Answer from the drawing. Dimensions are ordinates in mm from the lowest x, y and z of the part. Round coordinates to 2 decimals unless told otherwise and drop trailing zeros. Order: outer loops, then holes, each group sorted by start corner. A loop starts at its lowest first (then second) coordinate and runs counter-clockwise, first axis right, second up.
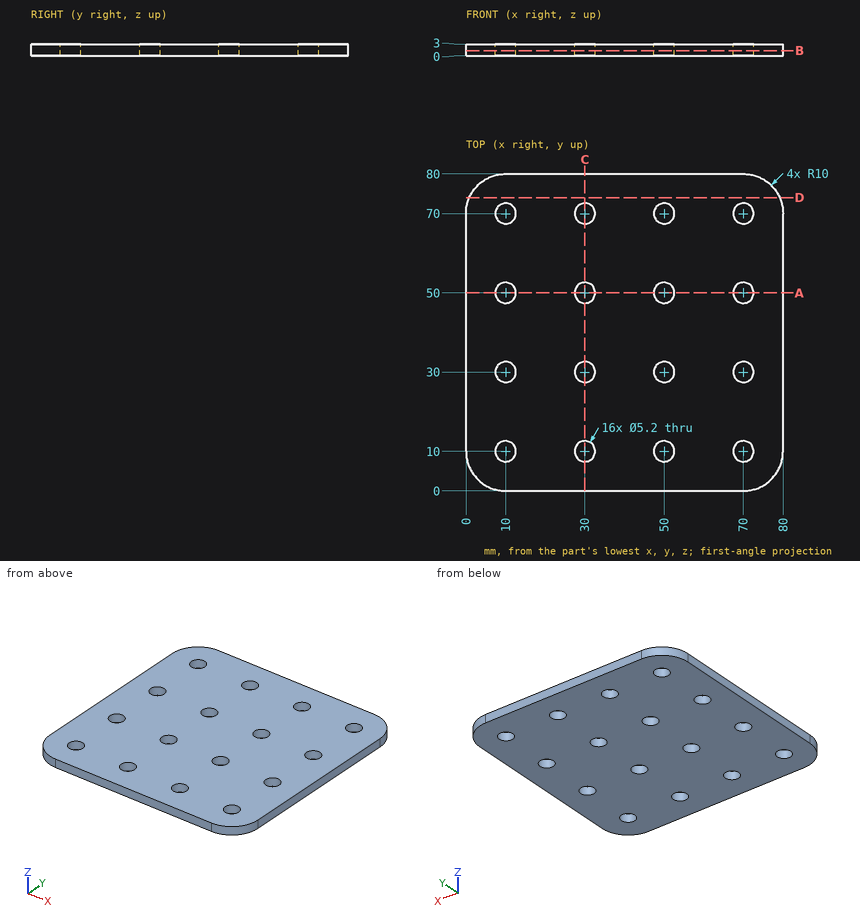
Q1. Straight lines are drawn through the part: probe 1 along Y at (x, z) = (50, 2.35); probe 2 along X at (y, z) = (31, 0.5). For each, find the intervals that lie inside material, in ascending order.
Outcome:
probe 1: y = 0 to 7.4, 12.6 to 27.4, 32.6 to 47.4, 52.6 to 67.4, 72.6 to 80
probe 2: x = 0 to 7.6, 12.4 to 27.6, 32.4 to 47.6, 52.4 to 67.6, 72.4 to 80
Q2. Flat-ended cylindrical pins translate along their axes: pin 1 (7 mm diameter, centred on x = 30, y = 30, fed in from -Z); pin 2 (3 mm diameter, centred on x = 10, y = 70, fed in from +Z) (3 decimals). Find the tip coordinate at first contact, or state that the pin passes through.
Outcome:
pin 1: stops at z = 0
pin 2: passes through
Q3. A cutting plane is placed at A-A, the plane y = 50. Give the vertices of the cut face in (x, z), plus the area to 3 significant figures.
Outcome:
outline: (0, 0) - (7.4, 0) - (7.4, 3) - (0, 3) - close; (12.6, 0) - (27.4, 0) - (27.4, 3) - (12.6, 3) - close; (32.6, 0) - (47.4, 0) - (47.4, 3) - (32.6, 3) - close; (52.6, 0) - (67.4, 0) - (67.4, 3) - (52.6, 3) - close; (72.6, 0) - (80, 0) - (80, 3) - (72.6, 3) - close
area: 178 mm2
Q4. A cutting plane is placed at B-B, the plane z = 1.3. Give the number of separate pieces and of enclosed holes in the cut face, plus the area to 3 significant figures.
Outcome:
separate pieces: 1
enclosed holes: 16
area: 5,970 mm2
Q5. A cutting plane is placed at D-D, the plane y = 74. Give the vertices of the cut face in (x, z).
Outcome:
outline: (0.83, 0) - (79.17, 0) - (79.17, 3) - (0.83, 3) - close
